Autodesk Inventor part; units mm, degrees
ref_plane "Work Plane1" through (-12.7, 25.4, 12.7) normal (-0.5774, -0.5774, -0.5774) x (0.7071, 0, -0.7071)
ref_plane "Work Plane2" through (12.7, 0, -12.7) normal (-0.5774, -0.5774, -0.5774) x (-0.7071, 0, 0.7071)
ref_plane "YZ Plane" through (0, 0, 0) normal (1, 0, 0) x (0, 1, 0)
sketch "Sketch1" plane through (0, 0, 0) normal (0, 1, 0) x (-1, 0, 0)
  line L0 (12.7, 12.7) -> (-12.7, 12.7)
  line L1 (-12.7, 12.7) -> (-12.7, -12.7)
  line L2 (-12.7, -12.7) -> (12.7, -12.7)
  line L3 (12.7, -12.7) -> (12.7, 12.7)
  point P0 (0, 0)
  dimension "d0" = 12.7
  dimension "d1" = 25.4
  dimension "d2" = 25.4
  dimension "d3" = 12.7
extrude "Extrusion1" add sketch "Sketch1" along normal blind 25.4
ref_plane "Work Plane1" through (-12.7, 25.4, 12.7) normal (-0.5774, -0.5774, -0.5774) x (0.7071, 0, -0.7071)
sketch "Sketch2" plane through (-12.7, 25.4, 12.7) normal (-0.5774, -0.5774, -0.5774) x (0.7071, 0, -0.7071)
  line L0 (-1.8052, -5.2104) -> (39.1986, -5.2104)
  line L1 (39.1986, -5.2104) -> (39.1986, 33.6585)
  line L2 (39.1986, 33.6585) -> (-1.8052, 33.6585)
  line L3 (-1.8052, 33.6585) -> (-1.8052, -5.2104)
  point P0 (17.9605, 20.739)
extrude "Extrusion2" cut sketch "Sketch2" against normal blind 25.4
ref_plane "Work Plane2" through (12.7, 0, -12.7) normal (-0.5774, -0.5774, -0.5774) x (-0.7071, 0, 0.7071)
sketch "Sketch3" plane through (12.7, 0, -12.7) normal (-0.5774, -0.5774, -0.5774) x (-0.7071, 0, 0.7071)
  line L0 (-4.9386, 41.2898) -> (46.8411, 41.2898)
  line L1 (46.8411, 41.2898) -> (46.8411, -12.9896)
  line L2 (46.8411, -12.9896) -> (-4.9386, -12.9896)
  line L3 (-4.9386, -12.9896) -> (-4.9386, 41.2898)
  point P0 (17.9605, 0)
extrude "Extrusion3" cut sketch "Sketch3" along normal blind 25.4
ref_plane "Work Plane3" through (-16.3662, 21.7338, 9.0338) normal (0.5774, 0.5774, 0.5774) x (0.7071, 0, -0.7071)
sketch "Sketch4" plane through (-16.3662, 21.7338, 9.0338) normal (0.5774, 0.5774, 0.5774) x (0.7071, 0, -0.7071)
  line L0 (44.1276, 17.5061) -> (-11.0494, 17.5061)
  line L1 (-11.0494, 17.5061) -> (-11.0494, -38.1771)
  line L2 (-11.0494, -38.1771) -> (44.1276, -38.1771)
  line L3 (44.1276, -38.1771) -> (44.1276, 17.5061)
  point P0 (17.9605, -20.739)
extrude "Extrusion4" cut sketch "Sketch4" against normal blind 25.4
properties part number "jimscube"
Work out the finished part from the listing and answer in its coordinate system (mm). Round coordinates to 2 decimals unless told otherwise and drop trailing zeros. Loops run counter-clockwise (first coordinate to the right, second up) from the corner with the lowest first, then second, coordinate; pieces in that order, holes last. Notation, with made-up numbers: (35, 55) - (48, 55) arc R17 cw to (48, 59) - close; hole circle Ø11 at (-16, 33.25). An arc over 180 degrees is marked (long way). One line per item, written item: value.
Q1. Straight lines are drawn through the part: probe 1 along Y at (x, z) = (5.25, -7); probe 2 along Y at (x, z) = (9.5, 3); probe 3 along Z at (x, y) = (5.75, 10.5). For each, find the intervals that lie inside material, in ascending order.
Check values:
probe 1: 16.15 to 25.4
probe 2: 1.9 to 12.9
probe 3: -1.85 to 9.15
Q2. Find section A-A on x = 9. Give the vertices of the cut face in (y, z).
Check values:
outline: (0, 5.4) - (18.1, -12.7) - (25.4, -12.7) - (25.4, -9) - (3.7, 12.7) - (0, 12.7) - close
Q3. Each of these flat-tipped pins is pushed along its axis until it touches: pin 1 Ø10 at (y, z) = (15, 10) entering from +X; pin 2 Ø12 at (y, z) = (21.5, 8) entering from +X; pin 3 Ø6 at (y, z) = (4.5, -2.5) entering from -X. Where does it stop, or does it pass through?
Check values:
pin 1: x = 7.47
pin 2: x = 4.38
pin 3: x = 8.16
Q4. Find section B-B on z = 7.5. Give the vertices of the cut face in (x, y).
Check values:
outline: (-12.7, 19.6) - (6.9, 0) - (12.7, 0) - (12.7, 5.2) - (-7.5, 25.4) - (-12.7, 25.4) - close
Q5. Find section C-C on y = 10. Give the vertices of the cut face in (x, z), and give its area (3 significant figures).
Check values:
outline: (-8.3, 12.7) - (12.7, -8.3) - (12.7, 2.7) - (2.7, 12.7) - close
area: 170 mm2
Q6. Find section D-D on x = -7.5. Give the vertices of the cut face in (y, z), and give its area (3 significant figures).
Check values:
outline: (9.2, 12.7) - (25.4, -3.5) - (25.4, 7.5) - (20.2, 12.7) - close
area: 118 mm2
